Can you work these out from the model? Positions are in its coordinate system, mm. A direction names the side the tool comes from. Give positions to 0.01 mm unless a question says otherwise; leave off trailing zeros. Loops run counter-clockwise (first coordinate to the right, second up) from the corner with the lowest first, then second, coordinate; pieces in that order, holes last.
from build123d import *

# Parameters (mm, degrees)
SKETCH_1_W          = 133
SKETCH_1_H          = 133
SKETCH_1_W_2        = 122.5
SKETCH_1_H_2        = 122.5
EXTRUDE_1_DEPTH     = 160
SKETCH_2_W          = 133
SKETCH_2_H          = 133
EXTRUDE_2_DEPTH     = 5
CHAMFER_1_SIZE      = 5
SKETCH_3_R          = 2.75
CUT_EXTRUDE_1_DEPTH = 5
CUT_EXTRUDE_2_DEPTH = 10


with BuildPart() as part:
    # 草图1 → 凸台-拉伸1 (new body)
    with BuildSketch(Plane(origin=(0, 0, 0), x_dir=(0, 0, -1), z_dir=(1, 0, 0))):
        Rectangle(SKETCH_1_W, SKETCH_1_H)
        Rectangle(SKETCH_1_W_2, SKETCH_1_H_2, mode=Mode.SUBTRACT)
    extrude(amount=EXTRUDE_1_DEPTH)

    # 草图2 → 凸台-拉伸2 (add)
    with BuildSketch(Plane(origin=(160, 0, 0), x_dir=(0, 0, -1), z_dir=(1, 0, 0))):
        Rectangle(SKETCH_2_W, SKETCH_2_H)
    extrude(amount=EXTRUDE_2_DEPTH)

    # 倒角1
    chamfer_1_edges = [part.edges().sort_by_distance(p)[0] for p in [
        (82.5, 66.5, 66.5),
        (82.5, 66.5, -66.5),
        (82.5, -66.5, -66.5),
        (82.5, -66.5, 66.5),
    ]]
    chamfer(chamfer_1_edges, length=CHAMFER_1_SIZE)

    # 草图3 → 切除-拉伸1 (cut)
    with BuildSketch(Plane(origin=(165, 0, 0), x_dir=(0, 0, -1), z_dir=(1, 0, 0))):
        with Locations((48, 48)):
            Circle(SKETCH_3_R)
        with Locations((48, -48)):
            Circle(SKETCH_3_R)
        with Locations((-48, -48)):
            Circle(SKETCH_3_R)
        with Locations((-48, 48)):
            Circle(SKETCH_3_R)
    extrude(amount=-CUT_EXTRUDE_1_DEPTH, mode=Mode.SUBTRACT)

    # 草图4 → 切除-拉伸2 (cut)
    with BuildSketch(Plane.XZ.offset(66.5)):
        with BuildLine():
            Line((40, 20), (0, 20))
            Line((0, 20), (0, -20))
            Line((0, -20), (40, -20))
            ThreePointArc((40, -20), (60, 0), (40, 20))
        make_face()
    extrude(amount=-CUT_EXTRUDE_2_DEPTH, mode=Mode.SUBTRACT)


solid = part.part
(1) Will these pins go through, and if not, where does the flat tip stop? P1, Ø2.5, axis at x = 22.5, y = -62.5, coming from the -Z side; P2, Ø5, axis at y = 46, z = -20.5, coming from the -X side; P3, Ø4.5, axis at y = 48, z = 48, coming from the -X side.
Returned:
P1: stops at z = -66.5
P2: stops at x = 160
P3: passes through
(2) Please list where these lines run through material, in increasing order: probe 1 along Y at (x, z) = (161, 48); probe 2 along Y at (x, z) = (61.5, 35).
Returned:
probe 1: y = -66.5 to -50.75, -45.25 to 45.25, 50.75 to 66.5
probe 2: y = -66.5 to -61.25, 61.25 to 66.5
(3) Which directions (+Z, -Z, +X, -X, +Y, -Y) give clear straight access to the entire face, cutting with the end or side of a thin tool? Please do faces 4 (the flat face through (20, -64, 20)), 5 (the flat face through (81, -1, -66.5)), 6 (the flat face through (79, 61.25, 1)).
Returned:
face 4: -X, -Y
face 5: -Z, +X, -X, +Y, -Y
face 6: -X
(4) Suppose I cut it at D-D on x = 23. List the corners of the cut face in (y, z) for me, plus the area to 3 significant figures.
Returned:
outline: (-66.5, -61.5) - (-61.5, -66.5) - (61.5, -66.5) - (66.5, -61.5) - (66.5, 61.5) - (61.5, 66.5) - (-61.5, 66.5) - (-66.5, 61.5) - (-66.5, 20) - (-61.25, 20) - (-61.25, 61.25) - (61.25, 61.25) - (61.25, -61.25) - (-61.25, -61.25) - (-61.25, -20) - (-66.5, -20) - close
area: 2,420 mm2
(5) Thinking about a two-plate mould opening in Y: for faces 1 (the flat face through (81, -1, 66.5)), 2 (the flat face through (81, -66.5, 1)), 3 (the flat face through (79, -61.25, 1)), which applies, pulls with the +Y half, pulls with the -Y half, needs draft (parallel to the pull), parting line crosses it, or undercut?
Returned:
face 1: needs draft
face 2: pulls with the -Y half
face 3: undercut
(6) Suppose I cut it at A-A on z = -48. List the corners of the cut face in (x, y) for me.
Returned:
outline: (0, -66.5) - (165, -66.5) - (165, -50.75) - (160, -50.75) - (160, -61.25) - (0, -61.25) - close; (0, 61.25) - (160, 61.25) - (160, 50.75) - (165, 50.75) - (165, 66.5) - (0, 66.5) - close; (160, -45.25) - (165, -45.25) - (165, 45.25) - (160, 45.25) - close
(7) Suppose I cut it at C-C on x = 120. List the corners of the cut face in (y, z) for me.
Returned:
outline: (-66.5, -61.5) - (-61.5, -66.5) - (61.5, -66.5) - (66.5, -61.5) - (66.5, 61.5) - (61.5, 66.5) - (-61.5, 66.5) - (-66.5, 61.5) - close; hole (-61.25, -61.25) - (61.25, -61.25) - (61.25, 61.25) - (-61.25, 61.25) - close
